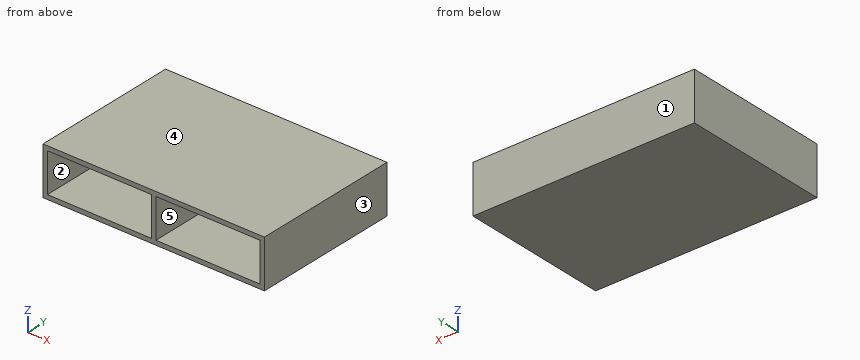
from build123d import *

# Parameters (mm, degrees)
F0_W     = 600
F0_H     = 130
F1_DEPTH = 400
F2_T     = -12
F3_W     = 12
F3_H     = 106
F4_DEPTH = 400


with BuildPart() as f1:
    # F0 (on Front) → F1 (new body)
    with BuildSketch(Plane.XZ):
        Rectangle(F0_W, F0_H)
    extrude(amount=-F1_DEPTH)

    # F2
    f2_openings = [f1.faces().sort_by_distance(p)[0] for p in [
        (0, 0, 0),
    ]]
    offset(amount=F2_T, openings=f2_openings)

    # F3 (on face) → F4 (join)
    with BuildSketch(Plane.XZ):
        Rectangle(F3_W, F3_H)
    extrude(amount=-F4_DEPTH)


solid = f1.part
Here's how the part is built. I have some questions about the finished solid (model axes, mm). Face numbers are marked on the shaded views. A direction names the side the tool comes from. Coordinates: 2 decimals unless noted, no trailing zeros. Order: outer loops, then holes, each group sorted by start corner. A loop starts at its lowest first (then second) coordinate and runs counter-clockwise, first axis right, second up. Notation, with made-up numbers: (14, 85.25) -> (62, 85.25) arc R28 ccw to (62, 115.25) -> close; hole circle Ø3 at (77, 56). An arc over 180 degrees is marked (long way). Answer in a Markdown table with one row per item.
(1) Thinking about a two-plate mould opening in X: for the marked faces 1, 2 and 3, which applies, +X half, -X half, draft (parallel to the pull), parting line (faces both ways), or undercut?
Answer key:
| item | result |
|---|---|
| face 1 | draft |
| face 2 | undercut |
| face 3 | +X half |
(2) Will this pin go through, and if not, where does the flat tip stop? pin 1 Ø4 at (x, z) = (-43, 14) entering from -Y.
Answer key:
| item | result |
|---|---|
| pin 1 | y = 388 |
(3) I want a section at C-C on x = -201.5. List the corners of the cut face in (y, z) for me.
Answer key:
| item | result |
|---|---|
| outline | (0, -65) -> (400, -65) -> (400, 65) -> (0, 65) -> (0, 53) -> (388, 53) -> (388, -53) -> (0, -53) -> close |
(4) On a 3-axis mill with a long thin cutter (end or side, diameter ignored), from which of +Z, -Z, +X, -X, +Y, -Y can I reach the whole of each face in a straight line? I mean the marked faces 4 and 5. Say none if no direction works.
Answer key:
| item | result |
|---|---|
| face 4 | +Z, +X, -X, +Y, -Y |
| face 5 | -Y |
(5) Please list where these lines run through material, in increasing order: probe 1 along X at (y, z) = (124.5, -7.5); probe 2 along Z at (x, y) = (144, 36); probe 3 along Y at (x, z) = (139.5, 12.5).
Answer key:
| item | result |
|---|---|
| probe 1 | -300 to -288, -6 to 6, 288 to 300 |
| probe 2 | -65 to -53, 53 to 65 |
| probe 3 | 388 to 400 |
(6) I want a section at B-B on z = -45. List the corners of the cut face in (x, y) for me, then the cut area to 3 significant figures.
Answer key:
| item | result |
|---|---|
| outline | (-300, 0) -> (-288, 0) -> (-288, 388) -> (-6, 388) -> (-6, 0) -> (6, 0) -> (6, 388) -> (288, 388) -> (288, 0) -> (300, 0) -> (300, 400) -> (-300, 400) -> close |
| area | 21,200 mm^2 |
(7) I want a section at A-A on y = 65. List the corners of the cut face in (x, z) for me.
Answer key:
| item | result |
|---|---|
| outline | (-300, -65) -> (300, -65) -> (300, 65) -> (-300, 65) -> close; hole (-288, -53) -> (-6, -53) -> (-6, 53) -> (-288, 53) -> close; hole (6, -53) -> (288, -53) -> (288, 53) -> (6, 53) -> close |
